from build123d import *

# Parameters (mm, degrees)
SKETCH1_W           = 251
SKETCH1_H           = 10
BOSS_EXTRUDE1_DEPTH = 10
SKETCH2_W           = 10
SKETCH2_H           = 10
CUT_EXTRUDE1_DEPTH  = 5
SKETCH4_W           = 10
SKETCH4_H           = 10
BOSS_EXTRUDE2_DEPTH = 40
CUT_EXTRUDE2_REACH  = 138.859
SKETCH5_R           = 5
SKETCH7_R           = 9
SKETCH7_R_2         = 5
BOSS_EXTRUDE3_DEPTH = 10


with BuildPart() as part:
    # Sketch1 → Boss-Extrude1 (new body)
    with BuildSketch(Plane.XY):
        with Locations((-125.5, 5)):
            Rectangle(SKETCH1_W, SKETCH1_H)
    extrude(amount=BOSS_EXTRUDE1_DEPTH)

    # Sketch2 → Cut-Extrude1 (cut)
    with BuildSketch(Plane.XY.offset(10)):
        with Locations((-188, 5)):
            Rectangle(SKETCH2_W, SKETCH2_H)
        with Locations((-63, 5)):
            Rectangle(SKETCH2_W, SKETCH2_H)
    extrude(amount=-CUT_EXTRUDE1_DEPTH, mode=Mode.SUBTRACT)

    # Sketch4 → Boss-Extrude2 (add)
    with BuildSketch(Plane(origin=(0, 0, 0), x_dir=(-1, 0, 0), z_dir=(0, 0, -1))):
        with Locations((125.5, 5)):
            Rectangle(SKETCH4_W, SKETCH4_H)
    extrude(amount=BOSS_EXTRUDE2_DEPTH)

    # Sketch5 → Cut-Extrude2 (cut, up to next)
    with BuildSketch(Plane.ZY.offset(130.5), mode=Mode.PRIVATE) as cut_extrude2_sk1:
        with Locations((-20, 5)):
            Circle(SKETCH5_R)
    cut_extrude2_tool1 = extrude(cut_extrude2_sk1.sketch, amount=-CUT_EXTRUDE2_REACH, mode=Mode.PRIVATE) & part.part
    add(cut_extrude2_tool1.solids().sort_by_distance((-130.5, 5, -20))[0], mode=Mode.SUBTRACT)


with BuildPart() as cut_extrude2_piece_1:
    # of the separate pieces the step leaves, piece 1, a body of its own (cut_extrude2_pieces)
    add(part.part.solids().sort_by_distance((0, 0, 0))[0])



with BuildPart() as cut_extrude2_piece_2:
    # of the separate pieces the step leaves, piece 2, a body of its own (cut_extrude2_pieces)
    add(part.part.solids().sort_by_distance((-120.5, 0, -40))[0])


with BuildPart() as cut_extrude2_piece_1_1:
    add(cut_extrude2_piece_1.part)

    add(cut_extrude2_piece_2.part)  # Boss-Extrude3 merges Cut-Extrude2 piece 2
    # Sketch7 → Boss-Extrude3 (add)
    with BuildSketch(Plane.ZY.offset(130.5)):
        with Locations((-20, 5)):
            Circle(SKETCH7_R)
        with Locations((-20, 5)):
            Circle(SKETCH7_R_2, mode=Mode.SUBTRACT)
    extrude(amount=-BOSS_EXTRUDE3_DEPTH)


solid = cut_extrude2_piece_1_1.part
Source: CAD feature listing. Evaluate the final solid. Frame: model axes, mm. A direction names the side the tool comes from. Round coordinates to 2 decimals unless told otherwise and drop trailing zeros. Loops run counter-clockwise (first coordinate to the right, second up) from the corner with the lowest first, then second, coordinate; pieces in that order, holes last. Notation, with made-up numbers: (65, -28.75) - (118, -28.75) arc R13 ccw to (118, -14.75) - close; hole circle Ø6 at (41, -29.5). An arc over 180 degrees is marked (long way). Write item = value, one per line. Start each with the question number.
(1) Set-up query: faces 1 (the face through (-126, 10, -34)), 2 (the face through (-192, 5, 0)), 3 (the face through (-68, 5, 8)), 4 (the face through (-120.5, 7, -15)). Return all of +Z, -Z, +X, -X, +Y, -Y with unobstructed straight access to the full face (end or side cutting, diameter ignored); none if empty.
(2) Section query B-B, the plane y = 5. Output: boundary loops of the cut face in (x, z), plus the area to 3 significant figures.
(3) Section query D-D, the plane z = -3.5. Output: boundary loops of the cut face in (x, y), plus the area to 3 significant figures.
(4) Section query C-C, the plane x = -82. Output: boundary loops of the cut face in (y, z), plus the area to 3 significant figures.
(5) Section query A-A, the plane z = -20. Output: boundary loops of the cut face in (x, y), plus the area to 3 significant figures.
(6) Pin query (flat end, axial travel): pin 1 (3 mm diameter, centred on x = -189.5, y = 2.5, fed in from +Z); pin 2 (1 mm diameter, centred on y = 6, z = 3.5, fed in from +X); pin 3 (5.5 mm diameter, centred on y = 6, z = -13.5, fed in from +X); pin 4 (1.5 mm diameter, centred on x = -36.5, y = 5, fed in from -Z). Return the tip coordinate at first contact, or that it passes through.
(7) Pull-direction query (Z, two-part tool) for faces 5 (the face through (-127, 10, 4)), 6 (the face through (-125.57, 9.77, -21.5)), 7 (the face through (-126, -4, -20)), 8 (the face through (-61, 5, 0)); classes: +Z half, -Z half, draft (parallel to the pull), parting line (faces both ways), or undercut.
(8) Ray query, line 1 along Z through (x, y) = (-123.25, 5); line 2 along Y through (x, z) = (-126, -20); line 3 along Y through (x, z) = (-213, 7.5). Return the intervals inside material, ascending. Write a range as from..to.
Conclusion:
q1.face_1 = -Z, +X, -X, +Y
q1.face_2 = -Z, -X, +Y, -Y
q1.face_3 = +Z, +Y, -Y
q1.face_4 = -Z, +X, +Y, -Y
q2.outline = (-251, 0) - (-130.5, 0) - (-130.5, -15) - (-120.5, -15) - (-120.5, 0) - (0, 0) - (0, 10) - (-58, 10) - (-58, 5) - (-68, 5) - (-68, 10) - (-183, 10) - (-183, 5) - (-193, 5) - (-193, 10) - (-251, 10) - close; (-130.5, -40) - (-120.5, -40) - (-120.5, -25) - (-130.5, -25) - close
q2.area = 2,710 mm2
q3.outline = (-130.5, 0) - (-120.5, 0) - (-120.5, 10) - (-130.5, 10) - close
q3.area = 100 mm2
q4.outline = (0, 0) - (10, 0) - (10, 10) - (0, 10) - close
q4.area = 100 mm2
q5.outline = (-130.5, -4) - (-120.5, -4) - (-120.5, 0) - (-130.5, 0) - close; (-130.5, 10) - (-120.5, 10) - (-120.5, 14) - (-130.5, 14) - close
q5.area = 80.0 mm2
q6.pin_1 = 5
q6.pin_2 = 0
q6.pin_3 = -120.5
q6.pin_4 = 0
q7.face_5 = draft
q7.face_6 = undercut
q7.face_7 = parting line
q7.face_8 = -Z half
q8.line_1 = -40..-25, -15..10
q8.line_2 = -4..0, 10..14
q8.line_3 = 0..10
